```python
from build123d import *

# Parameters (mm, degrees)
BOSS_EXTRUDE1_DEPTH = 12.7
SKETCH4_R           = 8.976739885
CUT_EXTRUDE1_DEPTH  = 120.43793735


with BuildPart() as part:
    # Sketch1 → Boss-Extrude1 (new body)
    with BuildSketch(Plane.XY):
        with BuildLine():
            Line((19.05, 51.687014291), (6.15479997, 102.487014291))
            ThreePointArc((6.15479997, 102.487014291), (0, 107.274664355), (-6.15479997, 102.487014291))
            Line((-6.15479997, 102.487014291), (-19.05, 51.687014291))
            Line((-19.05, 51.687014291), (-19.05, -117.222985709))
            Line((-19.05, -117.222985709), (19.05, -117.222985709))
            Line((19.05, -117.222985709), (19.05, 51.687014291))
        make_face()
    extrude(amount=BOSS_EXTRUDE1_DEPTH)

    # Sketch4 → Cut-Extrude1 (cut, through all)
    with BuildSketch(Plane(origin=(0, 0, 0), x_dir=(-1, 0, 0), z_dir=(0, 0, -1))):
        with Locations((0, 47.877014291)):
            Circle(SKETCH4_R)
    extrude(amount=-CUT_EXTRUDE1_DEPTH, mode=Mode.SUBTRACT)


solid = part.part
```
Design review of the part built by this model. Coordinates are the model's own, in mm. Give positions to 0.01 mm unless a question says otherwise; leave off trailing zeros. Order: outer loops, then holes, each group sorted by start corner. A loop starts at its lowest first (then second) coordinate and runs counter-clockwise, first axis right, second up. Notation, with made-up numbers: (24.5, -29.75) -> (59.5, -29.75) arc R9 ccw to (59.5, -13.75) -> close; hole circle Ø8 at (-3, 45.5). An arc over 180 degrees is marked (long way). Write each question's results on one line, items separated by ' | '. Start each with the question number.
Q1. Wall thickness on L1, parallel to Y at x = 0, z = 4; L2, parallel to Y at x = -0.5, z = 10; L3, parallel to X at y = 75.5, z = 12: over which ranges is each line inside the solid? List them lowest first. Write a range as from..to.
Q2. Add section B-B on z = 4.75. Give the boundary of the cut face in (x, y), and give its area (3 significant figures).
Q3. Add section D-D on y = 86.5. Give the boundary of the cut face in (x, z), and give its area (3 significant figures).
Q4. Add section A-A on x = 0. Give the boundary of the cut face in (y, z).
Q5. For pin 1 (3 mm diameter, centred on x = -1.5, y = -18, fed in from -Z), flat-tipped, find the tip position at first contact; note if it passes through.
Q6. Mouldability with a two-part tool opening along X and no side actions: class faces 1 (the flat face through (-12.512, 77.443, 6.261)), 2 (the cylindrical face through (7.12, 42.41, 6.26)), 3 (the cylindrical face through (0.118, 107.274, 6.261)) as +X half, -X half, draft (parallel to the pull), parting line (faces both ways), or undercut.
Q7. Add section C-C on x = -11.5. Give the boundary of the cut face in (y, z).
Found:
1) L1: y = -117.22..38.9, 56.85..107.27 | L2: y = -117.22..38.91, 56.84..107.25 | L3: x = -13.01..13.01
2) outline: (-19.05, -117.22) -> (19.05, -117.22) -> (19.05, 51.69) -> (6.15, 102.49) arc R6.35 ccw to (-6.15, 102.49) -> (-19.05, 51.69) -> close; hole circle Ø17.95 at (0, 47.88) | area: 7,510 mm2
3) outline: (-10.21, 0) -> (10.21, 0) -> (10.21, 12.7) -> (-10.21, 12.7) -> close | area: 259 mm2
4) outline: (-117.22, 0) -> (38.9, 0) -> (38.9, 12.7) -> (-117.22, 12.7) -> close; (56.85, 0) -> (107.27, 0) -> (107.27, 12.7) -> (56.85, 12.7) -> close
5) pin 1: stops at z = 0
6) face 1: -X half | face 2: undercut | face 3: parting line
7) outline: (-117.22, 0) -> (81.43, 0) -> (81.43, 12.7) -> (-117.22, 12.7) -> close
